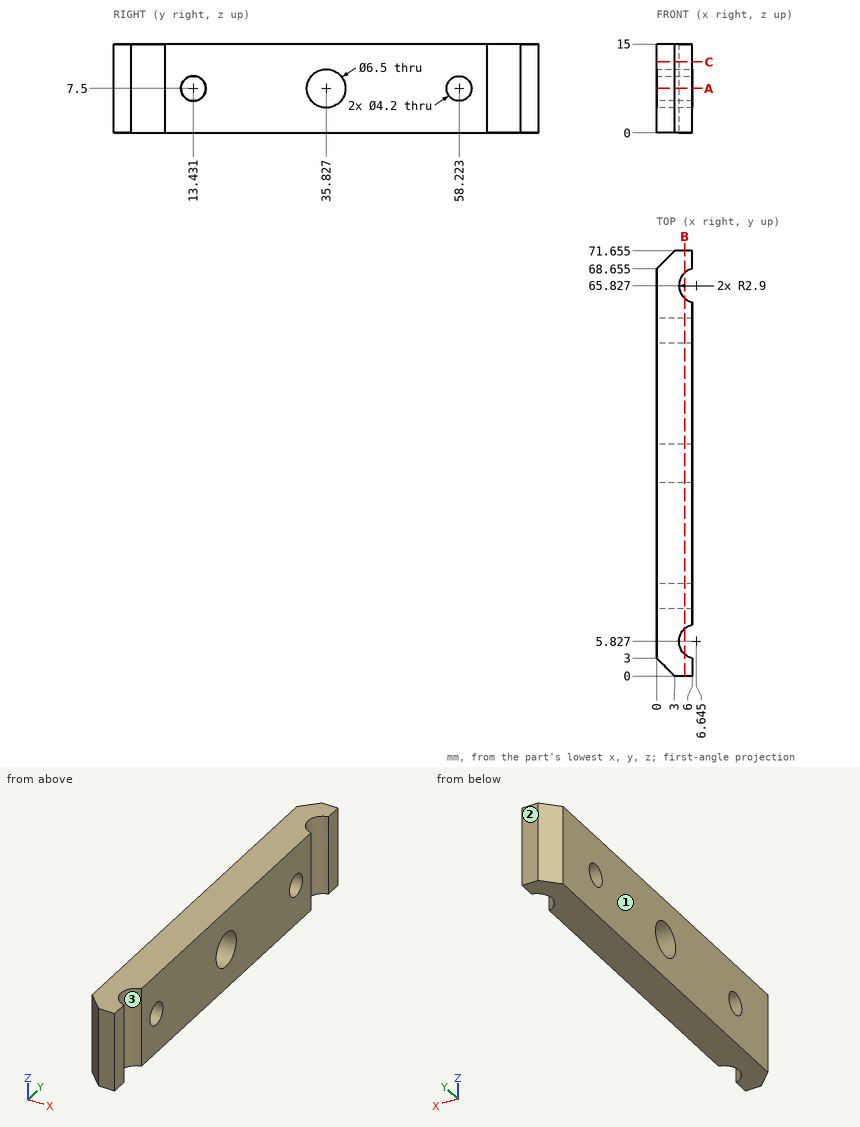
Answer from the drawing. Dimensions are ordinates in mm from the lowest x, y and z of the part. Coordinates: 2 decimals unless noted, no trailing zeros. Order: outer loops, then holes, each group sorted by start corner. A loop starts at its lowest first (then second) coordinate and runs counter-clockwise, first axis right, second up. Notation, with made-up numbers: (69, -9.5) - (83, -9.5) arc R22 cw to (83, 13.5) - close; hole circle Ø4 at (37.25, 58). An arc over 180 degrees is marked (long way). Put each result on its own line as item: value. Start each with the question number.
1) Find section A-A (z = 7.5). Give the vertices of the cut face in (x, y) (1 decimal).
2) For a pull along Y with two mould halves and no side action, classify the marked faces 1, 2 and 3 as released by +Y, released by -Y, zero draft, split by the parting line, or undercut.
3) Find section C-C (z = 12). Give the vertices of the cut face in (x, y) (1 decimal), plus the area to 3 significant figures.
4) Find section B-B (x = 4.7). State how many separate pieces and enclosed holes the cut face has, plus the area to 3 significant figures.
5) Flat-ended cylindrical pins translate along their axes: pin 1 (4 mm diameter, centred on y = 35.83, z = 7.5, fed in from -X); pin 2 (1 mm diameter, centred on x = 2.5, y = 59.5, fed in from -Z). Find the tip coordinate at first contact, or state that the pin passes through.
6) Find the intervals of material crossed by line 1 (Y direction, x = 3.2, z = 7.5) (1 decimal); line 2 (Y direction, x = 5.5, z = 6) (1 decimal); line 3 (Y direction, x = 5.5, z = 9.25) (1 decimal), in increasing order. Write a range as from..to.
Results list:
1. outline: (0, 3) - (3, 0) - (6, 0) - (6, 3) arc R2.9 cw to (6, 8.7) - (6, 11.3) - (0, 11.3) - close; (0, 15.5) - (6, 15.5) - (6, 32.6) - (0, 32.6) - close; (0, 39.1) - (6, 39.1) - (6, 56.1) - (0, 56.1) - close; (0, 60.3) - (6, 60.3) - (6, 63) arc R2.9 cw to (6, 68.7) - (6, 71.7) - (3, 71.7) - (0, 68.7) - close
2. face 1: zero draft
2. face 2: released by +Y
2. face 3: undercut
3. outline: (0, 3) - (3, 0) - (6, 0) - (6, 3) arc R2.9 cw to (6, 8.7) - (6, 63) arc R2.9 cw to (6, 68.7) - (6, 71.7) - (3, 71.7) - (0, 68.7) - close
3. area: 402 mm^2
4. separate pieces: 3
4. enclosed holes: 3
4. area: 885 mm^2
5. pin 1: passes through
5. pin 2: stops at z = 0
6. line 1: y = 0..11.3, 15.5..32.6, 39.1..56.1, 60.3..71.7
6. line 2: y = 0..3.2, 8.5..12, 14.9..32.9, 38.7..56.8, 59.7..63.2, 68.5..71.7
6. line 3: y = 0..3.2, 8.5..12.3, 14.6..33.1, 38.6..57.1, 59.4..63.2, 68.5..71.7
